Source: CAD feature listing. Evaluate the final solid. Frame: model axes, mm. Face numbers are marked on the shaded views. A direction names the side the tool comes from. Coordinates: 2 decimals unless noted, no trailing zeros. Write each loop counter-clockwise with the first axis right and the second up, starting at its lowest first coordinate (ties: lowest second). Pieces come first, ordered by that corner, then holes. Notation, with made-up numbers: M -30.5,-22 L -15.5,-22 A23 ccw -15.5,-2 Z; hole C 38.25,70.25 d4. An arc over 180 degrees is marked long. Answer as CSV lines item,"result". Start each with the question number.
1. Section C-C on z = 28. Return the cut outline in (x, y).
2. Section A-A on x = 0. Return the cut outline in (y, z), plus the area to 3 significant figures.
3. Section B-B on y = 0.5. Return the cut outline in (x, z), plus the area to 3 significant figures.
4. Section D-D on z = 2.5. Return the cut outline in (x, y).
5. Line query: probe 1 along Z at (x, y) = (0, 1.85); probe 2 along Z at (x, y) = (-3.5, -0.5); probe 3 along X at (y, z) = (0.6, 2.5). Output: solid intervals per line, ascending. Write a range as [from, to].
6. Reachability of the marked faces 1, 2 and 3 from +Z, -Z, +X, -X, +Y, -Y: full face, straight path, thin tool, end or side. Return the list, or none.
7. Contact query for flat-ended pins moving along their axis: pin 1 Ø3 at (x, z) = (0, 2.5) entering from -Y; pin 2 Ø1.5 at (y, z) = (-1.5, 33.5) entering from +X; pin 3 Ø2 at (y, z) = (1.5, 28) entering from -X. Output: stop coordinate, or through.
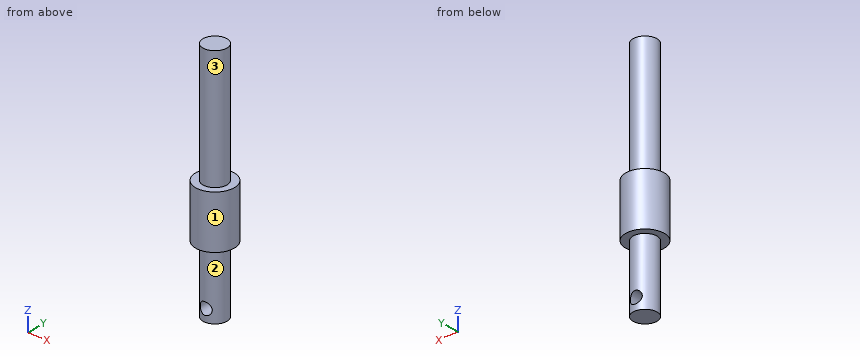
```python
from build123d import *

# Parameters (mm, degrees)
SKETCH1_R               = 2.5
BOSS_EXTRUDE1_DEPTH     = 13.8
BOSS_EXTRUDE3_START     = 13.8
SKETCH1_4_R             = 4
BOSS_EXTRUDE3_DEPTH     = 11
BOSS_EXTRUDE2_START     = 24.8
SKETCH1_3_R             = 2.5
BOSS_EXTRUDE2_DEPTH     = 24.9
SKETCH17_R              = 1.25
CUT_EXTRUDE1_DEPTH      = 5
CUT_EXTRUDE1_DEPTH_BACK = 5


with BuildPart() as part:
    # Sketch1 → Boss-Extrude1 (new body)
    with BuildSketch(Plane.XY):
        Circle(SKETCH1_R)
    extrude(amount=BOSS_EXTRUDE1_DEPTH)

    # Sketch1<4> → Boss-Extrude3 (add)
    with BuildSketch(Plane.XY.offset(BOSS_EXTRUDE3_START)):
        Circle(SKETCH1_4_R)
    extrude(amount=BOSS_EXTRUDE3_DEPTH)

    # Sketch1<3> → Boss-Extrude2 (add)
    with BuildSketch(Plane.XY.offset(BOSS_EXTRUDE2_START)):
        Circle(SKETCH1_3_R)
    extrude(amount=BOSS_EXTRUDE2_DEPTH)

    # Sketch17 → Cut-Extrude1 (cut, two sides)
    with BuildSketch(Plane(origin=(0, 0, 0), x_dir=(1, 0, 0), z_dir=(0, 1, 0))) as cut_extrude1_sk:
        with Locations((0, -2.5)):
            Circle(SKETCH17_R)
    extrude(amount=CUT_EXTRUDE1_DEPTH, mode=Mode.SUBTRACT)
    extrude(cut_extrude1_sk.sketch, amount=-CUT_EXTRUDE1_DEPTH_BACK, mode=Mode.SUBTRACT)


solid = part.part
```
Values:
1,outline,"C 0,0 d5"
2,outline,"M -4,13.8 L -2.5,13.8 L -2.5,3.75 L 2.5,3.75 L 2.5,13.8 L 4,13.8 L 4,24.8 L 2.5,24.8 L 2.5,49.7 L -2.5,49.7 L -2.5,24.8 L -4,24.8 Z; M -2.5,0 L 2.5,0 L 2.5,1.25 L -2.5,1.25 Z"
2,area,"269 mm²"
3,outline,"M -3.97,13.8 L -2.45,13.8 L -2.45,0 L 2.45,0 L 2.45,13.8 L 3.97,13.8 L 3.97,24.8 L 2.45,24.8 L 2.45,49.7 L -2.45,49.7 L -2.45,24.8 L -3.97,24.8 Z; hole C 0,2.5 d2.5"
3,area,"272 mm²"
4,outline,"M -1.25,-2.17 L -1.25,2.17 A2.5 ccw Z; M 1.25,-2.17 A2.5 ccw 1.25,2.17 Z"
5,probe 1,"[0, 1.25], [3.75, 49.7]"
5,probe 2,"[13.8, 24.8]"
5,probe 3,"[-2.43, -1.25], [1.25, 2.43]"
6,face 1,"+Z, -Z"
6,face 2,"-Z"
6,face 3,"+Z"
7,pin 1,"y = -2.5"
7,pin 2,"x = 2.38"
7,pin 3,"x = -2.45"
